Build history of the part. All positions in model axes, mm. A direction names the side the tool comes from. Round coordinates to 2 decimals unless told otherwise and drop trailing zeros. Write each loop counter-clockwise with the first axis right and the second up, starting at its lowest first coordinate (ties: lowest second). Pieces come first, ordered by that corner, then holes. Notation, with made-up numbers: (-39.75, 81) -> (-30.75, 81) arc R13 cw to (-30.75, 103) -> close; hole circle Ø10 at (-31.5, 2). An arc over 180 degrees is marked (long way). Return JSON: item names as keys, results as strings.
from build123d import *

# Parameters (mm, degrees)
BOSS_EXTRUDE1_DEPTH            = 24
CUT_EXTRUDE1_DEPTH             = 25
SKETCH3_W                      = 7.55
SKETCH3_H                      = 24
F_4_5_4_5_DIAMETER_HOLE1_D     = 4.5
F_4_5_4_5_DIAMETER_HOLE1_DEPTH = 6


with BuildPart() as part:
    # Sketch1 → Boss-Extrude1 (new body)
    with BuildSketch(Plane(origin=(0, 24, 0), x_dir=(1, 0, 0), z_dir=(0, 1, 0))):
        with BuildLine():
            Line((0, 0), (47, 0))
            Line((47, 0), (47, 6))
            Line((47, 6), (38.5, 6))
            ThreePointArc((38.5, 6), (35.307693119, 7.131854655), (33.541354656, 10.021831577))
            ThreePointArc((33.541354656, 10.021831577), (23.505747016, 20.045434485), (13.49594739, 9.996059012))
            ThreePointArc((13.49594739, 9.996059012), (11.698748894, 7.121907302), (8.5, 6))
            Line((8.5, 6), (0, 6))
            Line((0, 6), (0, 0))
        make_face()
    extrude(amount=-BOSS_EXTRUDE1_DEPTH)

    # Sketch2 → Cut-Extrude1 (cut, through all)
    with BuildSketch(Plane.XZ):
        with BuildLine():
            Line((24.018633311, 0), (23.018633311, 0))
            Line((23.018633311, 0), (23.018633311, -2.489295869))
            ThreePointArc((23.018633311, -2.489295869), (23.518633311, -2.472721384), (24.018633311, -2.489295869))
            Line((24.018633311, -2.489295869), (24.018633311, 0))
        make_face()
    extrude(amount=-CUT_EXTRUDE1_DEPTH, mode=Mode.SUBTRACT)

    # Sketch3 → Cut-Revolve1 (revolve, cut)
    with BuildSketch(Plane(origin=(0, 0, -10.022721384), x_dir=(-1, 0, 0), z_dir=(0, 0, -1))):
        with Locations((-27.293633311, 12)):
            Rectangle(SKETCH3_W, SKETCH3_H)
    revolve(axis=Axis((23.518633311, 0, -10.022721384), (0, 1, 0)), mode=Mode.SUBTRACT)

    # Ø4.5 (4.5) Diameter Hole1
    with Locations(Plane(origin=(0, 0, -6), x_dir=(-1, 0, 0), z_dir=(0, 0, -1))):
        with Locations((-41.037266621, 12), (-6, 12)):
            Hole(F_4_5_4_5_DIAMETER_HOLE1_D / 2, depth=F_4_5_4_5_DIAMETER_HOLE1_DEPTH)


solid = part.part
Q1. Saw through at A-A on y = 12. List the corners of the cut face in (x, z).
Verdict:
{"outline": "(0, -6) -> (3.75, -6) -> (3.75, 0) -> (0, 0) -> close; (8.25, -6) -> (8.5, -6) arc R5.12 cw to (13.5, -10) arc R10.02 ccw to (33.54, -10.02) arc R5.07 cw to (38.5, -6) -> (38.79, -6) -> (38.79, 0) -> (24.02, 0) -> (24.02, -2.49) arc R7.55 cw (long way) to (23.02, -2.49) -> (23.02, 0) -> (8.25, 0) -> close; (43.29, -6) -> (47, -6) -> (47, 0) -> (43.29, 0) -> close"}
Q2. Saw through at B-B on x = 6. List the corners of the cut face in (y, z), then the cut area to 3 significant figures.
Verdict:
{"outline": "(0, -6) -> (9.75, -6) -> (9.75, 0) -> (0, 0) -> close; (14.25, -6) -> (24, -6) -> (24, 0) -> (14.25, 0) -> close", "area": "117 mm²"}
Q3. Wall check: L1, parallel to Y at x = 6, z = -4.3; L2, parallel to X at y = 19.5, z = -1; L3, parallel to X at y = 8.5, z = -16.5. Give the ranges that are in metal, low to high.
Verdict:
{"L1": "y = 0 to 9.75, 14.25 to 24", "L2": "x = 0 to 23.02, 24.02 to 47", "L3": "x = 15.87 to 19.64, 27.4 to 31.17"}
Q4. 3-axis set-ups, long thin cutter, end or side, ignore diameter. For faces 5 (the cylindrical face through (7.21, 13.897, -2.958)), 6 (the flat face through (24.019, 12, -1)), 7 (the flat face through (3, 12, -6)): which of +Z, -Z, +X, -X, +Y, -Y reach the whole face in a straight line?
Verdict:
{"face 5": "+Z, -Z", "face 6": "+Z, +Y, -Y", "face 7": "-Z, -X, +Y, -Y"}
Q5. Two-plate mould, pull along X, no slides. Class faces 1 (the flat face through (23.019, 12, -1)), 2 (the cylindrical face through (43.18, 12.68, -2.96)), 3 (the flat face through (44, 12, -6)), 4 (the cylindrical face through (35.35, 12.17, -7.1)): +X half, -X half, draft (parallel to the pull), parting line (faces both ways), or undercut.
Verdict:
{"face 1": "undercut", "face 2": "undercut", "face 3": "draft", "face 4": "+X half"}
Q6. Pin check, flat tips, straight feed: pin 1 Ø6 at (x, y) = (6, 12) entering from -Z; pin 2 Ø1.5 at (y, z) = (20.5, -9.5) entering from -X; pin 3 Ø3.5 at (x, y) = (41.04, 12) entering from -Z; pin 4 Ø1.5 at (y, z) = (9.5, -16.5) entering from +X. Stop position of each tip, or through.
Verdict:
{"pin 1": "stops at z = -6.02", "pin 2": "stops at x = 13.04", "pin 3": "passes through", "pin 4": "stops at x = 31.74"}
Q7. Saw through at D-D on y = 15.5. List the corners of the cut face in (x, z), then the cut area to 3 significant figures.
Verdict:
{"outline": "(0, -6) -> (8.5, -6) arc R5.12 cw to (13.5, -10) arc R10.02 ccw to (33.54, -10.02) arc R5.07 cw to (38.5, -6) -> (47, -6) -> (47, 0) -> (24.02, 0) -> (24.02, -2.49) arc R7.55 cw (long way) to (23.02, -2.49) -> (23.02, 0) -> (0, 0) -> close", "area": "349 mm²"}
Q8. Saw through at C-C on z = -17. List the corners of the cut face in (x, y).
Verdict:
{"outline": "(16.32, 0) -> (20.63, 0) -> (20.63, 24) -> (16.32, 24) -> close; (26.4, 0) -> (30.71, 0) -> (30.71, 24) -> (26.4, 24) -> close"}
